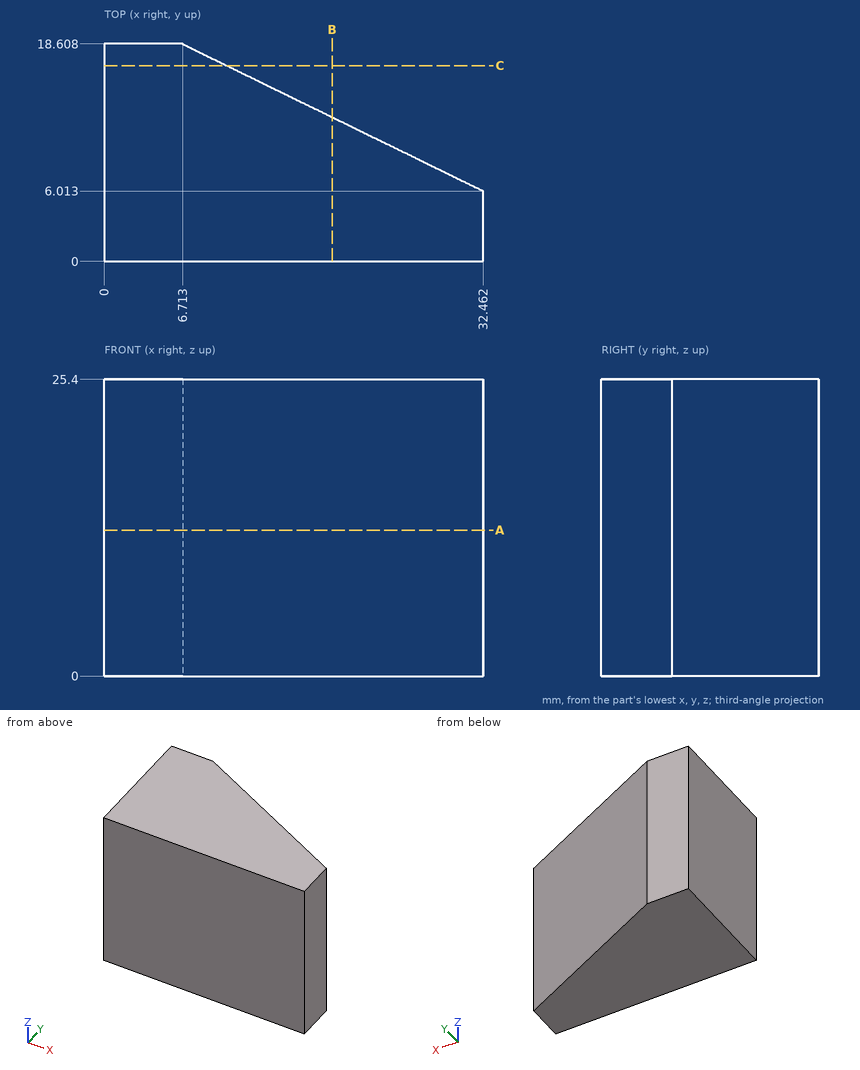
Print and shaded views of the part. All mm, measured from the part's lowest x, y and z. Round coordinates to 2 decimals unless told otherwise and drop trailing zeros. Order: outer loops, then holes, each group sorted by start corner. A loop starts at its lowest first (then second) coordinate and runs counter-clockwise, first axis right, second up. Notation, with made-up numbers: (34, 16) - (67, 16) arc R15 ccw to (67, 28) - close; hole circle Ø1 at (23, -22). An arc over 180 degrees is marked (long way). Use a Markdown table: item, result.
1) Saw through at B-B on x = 19.5. Write the cut outline in (y, z).
Recorded:
| item | result |
|---|---|
| outline | (0, 0) - (12.35, 0) - (12.35, 25.4) - (0, 25.4) - close |
2) Saw through at A-A on z = 12.5. Write the cut outline in (x, y).
Recorded:
| item | result |
|---|---|
| outline | (0, 0) - (32.46, 0) - (32.46, 6.01) - (6.71, 18.61) - (0, 18.61) - close |
3) Wall check: L1, parallel to X at y = 8.75, z = 19.25 (1 decimal); L2, parallel to X at y = 6.5, z = 3 (1 decimal); L3, parallel to Y at x = 12, z = 19.75. Give the ranges that are in metal, low to high.
Recorded:
| item | result |
|---|---|
| L1 | x = 0 to 26.9 |
| L2 | x = 0 to 31.5 |
| L3 | y = 0 to 16.02 |
4) Saw through at C-C on y = 16.75. Write the cut outline in (x, z), and give its area (3 significant figures).
Recorded:
| item | result |
|---|---|
| outline | (0, 0) - (10.51, 0) - (10.51, 25.4) - (0, 25.4) - close |
| area | 267 mm² |
5) Flat gauge pins, fed straight in: pin 1 Ø1 at (x, z) = (22, 15.5) entering from -Y; pin 2 Ø2 at (y, z) = (16.5, 9) entering from +X (1 decimal); pin 3 Ø6 at (x, z) = (28, 19.5) entering from +Y. Where does each tip first touch, or does it go through?
Recorded:
| item | result |
|---|---|
| pin 1 | stops at y = 0 |
| pin 2 | stops at x = 13.1 |
| pin 3 | stops at y = 9.66 |
